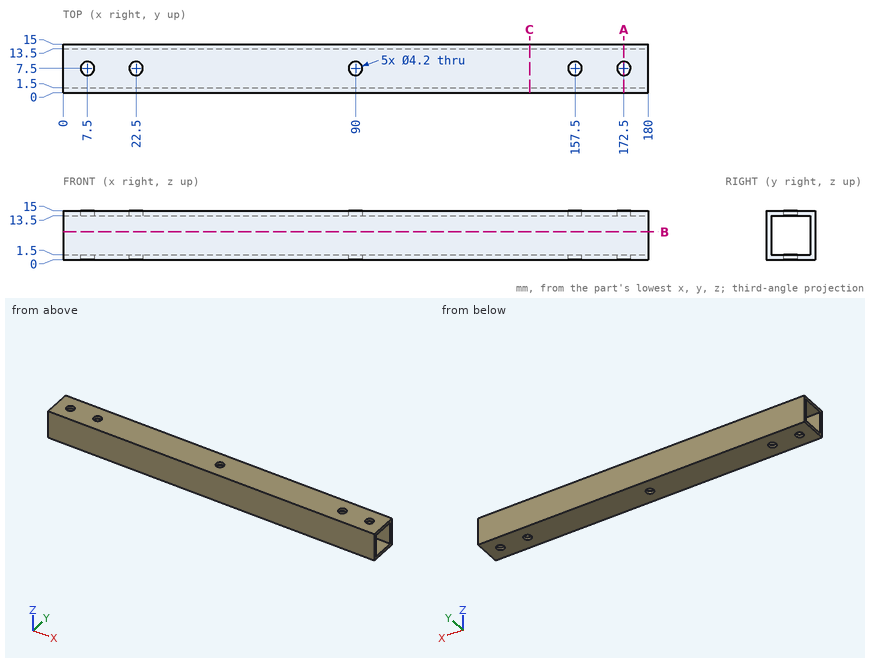
Answer from the drawing. Dimensions are ordinates in mm from the lowest x, y and z of the part. Coordinates: 2 decimals unless noted, no trailing zeros. Write each loop counter-clockwise with the first axis right and the second up, starting at its lowest first coordinate (ties: lowest second). Pieces come first, ordered by that corner, then holes. Notation, with made-up numbers: (23.5, 86) - (67.5, 86) arc R35 ccw to (67.5, 123) - close; hole circle Ø2 at (14, -8). An arc over 180 degrees is marked (long way). Return JSON: item names as keys, results as strings. Group by question number.
Q1. The part is cut by section C-C on x = 143.5. Write down the section's boundary in (y, z).
Q2. Find the intervals of material crossed by line 1 along Z through (x, y) = (22, 4); line 2 along Y through (x, z) = (157.5, 0.8), in increasing order. Write a range as [from, to].
Q3. The part is cut by section B-B on z = 8.5. Write down the section's boundary in (x, y).
Q4. A flat-ended cylindrical pin translates along its axis: pin 1 Ø2.5 at (x, y) = (90, 7.5) entering from -Z. Find the tip coordinate at first contact, or state that the pin passes through.
Q5. The part is cut by section A-A on x = 172.5. Write down the section's boundary in (y, z), and give its area (3 significant figures).
Evaluation:
{
 "1": {"outline": "(0, 0) - (15, 0) - (15, 15) - (0, 15) - close; hole (1.5, 1.5) - (13.5, 1.5) - (13.5, 13.5) - (1.5, 13.5) - close"},
 "2": {"line 1": "z = [0, 1.5], [13.5, 15]", "line 2": "y = [0, 5.4], [9.6, 15]"},
 "3": {"outline": "(0, 0) - (180, 0) - (180, 1.5) - (0, 1.5) - close; (0, 13.5) - (180, 13.5) - (180, 15) - (0, 15) - close"},
 "4": {"pin 1": "passes through"},
 "5": {"outline": "(0, 0) - (5.4, 0) - (5.4, 1.5) - (1.5, 1.5) - (1.5, 13.5) - (5.4, 13.5) - (5.4, 15) - (0, 15) - close; (9.6, 0) - (15, 0) - (15, 15) - (9.6, 15) - (9.6, 13.5) - (13.5, 13.5) - (13.5, 1.5) - (9.6, 1.5) - close", "area": "68.4 mm2"}
}
